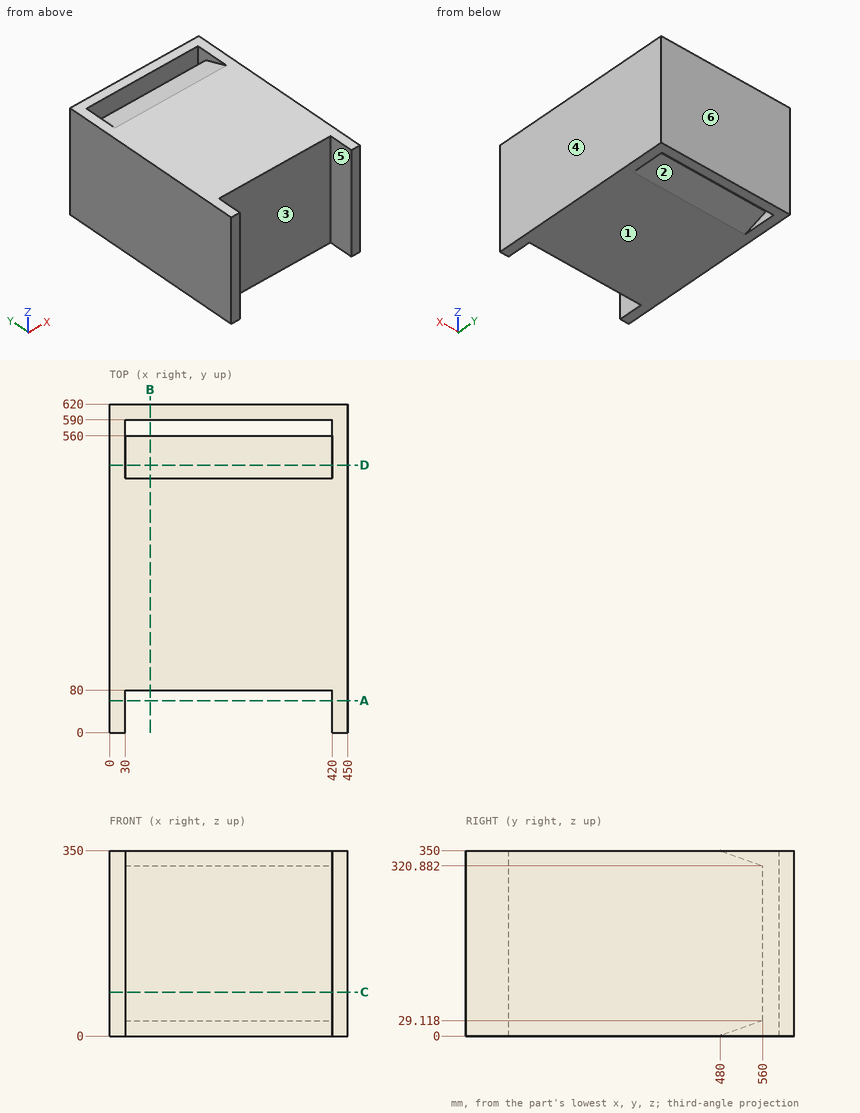
Geometry check sheet. Reference: drawing and pictorial views, mm from the part's lowest x, y, z. A direction names the side the tool comes from. Give positions to 0.01 mm unless a question says otherwise; leave off trailing zeros. Write each loop counter-clockwise with the first axis right and the second up, starting at its lowest first coordinate (ties: lowest second). Pieces come first, ordered by that corner, then holes. Notation, with made-up numbers: M 44,-11.75 L 74,-11.75 A6 ccw 74,-4.75 Z; hole C -34.5,24.5 d2. An arc over 180 degrees is marked long. Use CSV: the item, a comma, the result in double quotes.
1) Cross-section at D-D (y = 504.5). Enter the section's corners in (x, z), plus the area to 3 significant figures.
Final values:
outline,"M 0,0 L 30,0 L 30,8.92 L 420,8.92 L 420,0 L 450,0 L 450,350 L 420,350 L 420,341.08 L 30,341.08 L 30,350 L 0,350 Z"
area,"151,000 mm²"
2) Go/stop test with flat-tipped pins: pin 1 Ø4 at (x, z) = (276, 245.5) entering from -Y; pin 2 Ø2 at (x, y) = (357.5, 542.5) entering from -Z. Record where each tip stops, or that it passes through.
Final values:
pin 1,"y = 80"
pin 2,"z = 22.38"
3) Cross-section at A-A (y = 60). Enter the section's corners in (x, z).
Final values:
outline,"M 0,0 L 30,0 L 30,350 L 0,350 Z; M 420,0 L 450,0 L 450,350 L 420,350 Z"
4) Access from +Z, -Z, +X, -X, +Y, -Y to the whole of each face (thin tool, end or side, straight path). Record for the marked faces 1, 2 and 3.
Final values:
face 1,"-Z, +X, -X, +Y, -Y"
face 2,"-Z"
face 3,"+Z, -Z, -Y"
5) Cross-section at C-C (z = 83). Enter the section's corners in (x, y).
Final values:
outline,"M 0,0 L 30,0 L 30,80 L 420,80 L 420,0 L 450,0 L 450,620 L 0,620 Z; hole M 30,560 L 420,560 L 420,590 L 30,590 Z"
6) Release check for a two-part mould opening along X. For the marked faces 4, 5 and 6 record: released by +X, released by -X, zero draft, split by the parting line, or undercut.
Final values:
face 4,"released by +X"
face 5,"undercut"
face 6,"zero draft"
7) Cross-section at B-B (x = 76.5). Enter the section's corners in (y, z).
Final values:
outline,"M 80,0 L 480,0 L 560,29.12 L 560,320.88 L 480,350 L 80,350 Z; M 590,0 L 620,0 L 620,350 L 590,350 Z"
8) Material ranges on line 1 along Y through (x, z) = (112, 110); line 2 along X through (y, z) = (563, 102); line 3 along Z through (x, y) = (299.5, 531), recorded low to high.
Final values:
line 1,"80 to 560, 590 to 620"
line 2,"0 to 30, 420 to 450"
line 3,"18.56 to 331.44"
